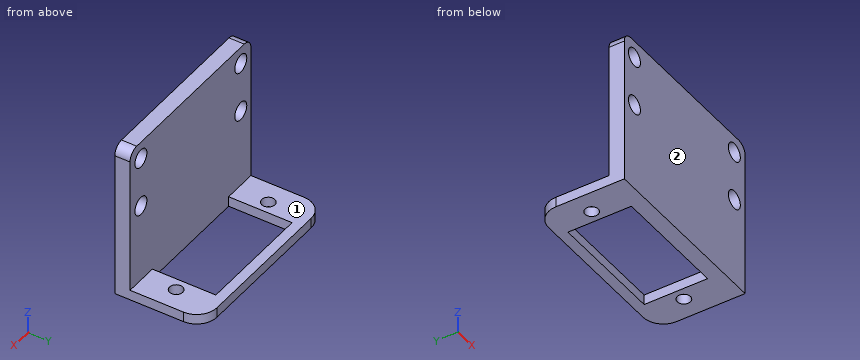
from build123d import *

# Parameters (mm, degrees)
SKETCH1_W            = 36.3
SKETCH1_H            = 16.5
SKETCH1_W_2          = 22.89999
SKETCH1_H_2          = 12.5
BOSS_EXTRUDE1_DEPTH  = 2
FILLET1_R            = 4
M2_CLEARANCE_HOLE1_D = 2.6
SKETCH4_W            = 36.3
SKETCH4_H            = 3
BOSS_EXTRUDE2_DEPTH  = 29
SKETCH4_2_W          = 36.3
SKETCH4_2_H          = 3
BOSS_EXTRUDE3_DEPTH  = 2
FILLET2_R            = 2
M3_CLEARANCE_HOLE1_D = 3.6


with BuildPart() as part:
    # Sketch1 → Boss-Extrude1 (new body)
    with BuildSketch(Plane.XY):
        with Locations((17.65, 8.830531887)):
            Rectangle(SKETCH1_W, SKETCH1_H)
        with Locations((17.65, 8.830531887)):
            Rectangle(SKETCH1_W_2, SKETCH1_H_2, mode=Mode.SUBTRACT)
    extrude(amount=BOSS_EXTRUDE1_DEPTH)

    # Fillet1
    fillet1_edges = [part.edges().sort_by_distance(p)[0] for p in [
        (-0.5, 17.080531887, 1),
        (35.8, 17.080531887, 1),
    ]]
    fillet(fillet1_edges, radius=FILLET1_R)

    # M2 Clearance Hole1 (through all)
    with Locations(Plane.XY.offset(2)):
        with Locations((31.5, 8.830531887), (3.8, 8.830531887)):
            Hole(M2_CLEARANCE_HOLE1_D / 2)

    # Sketch4 → Boss-Extrude2 (add)
    with BuildSketch(Plane.XY.offset(2)):
        with Locations((17.65, 1.080531887)):
            Rectangle(SKETCH4_W, SKETCH4_H)
    extrude(amount=BOSS_EXTRUDE2_DEPTH)

    # Sketch4<2> → Boss-Extrude3 (add)
    with BuildSketch(Plane.XY.offset(2)):
        with Locations((17.65, 1.080531887)):
            Rectangle(SKETCH4_2_W, SKETCH4_2_H)
    extrude(amount=-BOSS_EXTRUDE3_DEPTH)

    # Fillet2
    fillet2_edges = [part.edges().sort_by_distance(p)[0] for p in [
        (-0.5, 1.080531887, 31),
        (35.8, 1.080531887, 31),
    ]]
    fillet(fillet2_edges, radius=FILLET2_R)

    # M3 Clearance Hole1 (through all)
    with Locations(Plane(origin=(0, 2.580531887, 0), x_dir=(1, 0, 0), z_dir=(0, 1, 0))):
        with Locations((2.550005, -17.6), (2.550005, -27.6), (32.550005, -17.6), (32.550005, -27.6)):
            Hole(M3_CLEARANCE_HOLE1_D / 2)


solid = part.part
Source: CAD feature listing. Evaluate the final solid. Frame: model axes, mm. Face numbers are marked on the shaded views. A direction names the side the tool comes from. Round coordinates to 2 decimals unless told otherwise and drop trailing zeros. Order: outer loops, then holes, each group sorted by start corner. A loop starts at its lowest first (then second) coordinate and runs counter-clockwise, first axis right, second up. Notation, with made-up numbers: (-32, 28.25) - (-2, 28.25) arc R13 ccw to (-2, 33.25) - close; hole circle Ø4 at (13, -37.5). An arc over 180 degrees is marked (long way). Use a Markdown table: item, result. Add a question column.
1. Section query B-B (z = 17.6). Return the cut outline in (x, y).
2. First-contact query: pin 1 (4 mm diameter, centred on x = 32.55, z = 27.6, fed in from +Y); pin 2 (4 mm diameter, centred on x = 3.8, y = 8.83, fed in from +Z). Flat tips, straight axial feed; report the tip coordinate or a pass-through.
3. Line query: probe 1 along X at (y, z) = (1.75, 17.6); probe 2 along X at (y, z) = (2, 18.5); probe 3 along Y at (x, z) = (26.5, 8.5). Output: solid intervals per line, ascending.
4. Section query D-D (z = 7). Return the cut outline in (x, y).
5. Section query A-A (y = 6.75). Return the cut outline in (x, z).
6. Section query C-C (x = 24). Return the cut outline in (y, z), then the cut area to 3 significant figures.
7. Set-up query: the marked faces 1 and 2. Return all of +Z, -Z, +X, -X, +Y, -Y with unobstructed straight access to the full face (end or side cutting, diameter ignored); none if empty.
Derived:
| question | item | result |
|---|---|---|
| 1 | outline | (-0.5, -0.42) - (0.75, -0.42) - (0.75, 2.58) - (-0.5, 2.58) - close; (4.35, -0.42) - (30.75, -0.42) - (30.75, 2.58) - (4.35, 2.58) - close; (34.35, -0.42) - (35.8, -0.42) - (35.8, 2.58) - (34.35, 2.58) - close |
| 2 | pin 1 | y = 2.58 |
| 2 | pin 2 | z = 2 |
| 3 | probe 1 | -0.5 to 0.75, 4.35 to 30.75, 34.35 to 35.8 |
| 3 | probe 2 | -0.5 to 0.99, 4.11 to 30.99, 34.11 to 35.8 |
| 3 | probe 3 | -0.42 to 2.58 |
| 4 | outline | (-0.5, -0.42) - (35.8, -0.42) - (35.8, 2.58) - (-0.5, 2.58) - close |
| 5 | outline | (-0.5, 0) - (6.2, 0) - (6.2, 2) - (-0.5, 2) - close; (29.1, 0) - (35.8, 0) - (35.8, 2) - (29.1, 2) - close |
| 6 | outline | (-0.42, 0) - (2.58, 0) - (2.58, 31) - (-0.42, 31) - close; (15.08, 0) - (17.08, 0) - (17.08, 2) - (15.08, 2) - close |
| 6 | area | 97.0 mm2 |
| 7 | face 1 | +Z, +X, -X, +Y |
| 7 | face 2 | +Z, -Z, +X, -X, -Y |
